Here's how the part is built. I have some questions about the finished solid (model axes, mm). A direction names the side the tool comes from. Give positions to 0.01 mm unless a question says otherwise; leave off trailing zeros. Loops run counter-clockwise (first coordinate to the right, second up) from the corner with the lowest first, then second, coordinate; pieces in that order, holes last.
Q1. For faces 1 (the face through (-0.95, 0.78, -126.09)), 2 (the face through (-0.91, 0.78, -102.55)), which set-ups out of +Z, -Z, +X, -X, +Y, -Y let a thin tool reach every point of the face, with its end or its side?
Q2. If we section it at B-B (x = -76.2): Please give me the cut outline in (y, z), plus the area to 3 significant figures.
Q3. We'd pull the mould along X, two halves only. Please class faces 3 (the face through (-42.125, 0.805, -5.834)), 4 (the face through (-54, 1.588, -63)), 5 (the face through (-87.95, 0.78, -0.91)), 6 (the face through (-37.19, 0.78, -100.65)): +X half, -X half, draft (parallel to the pull), parting line (faces both ways), or undercut.
Q4. If we section it at A-A (z = -63.5): Please give me the cut outline in (x, y).
Q5. I need wall thicknesses on line 1 (Z direction, x = -44.45, y = 0.9); line 2 (X direction, y = 1.2, z = -12.7); line 3 (X direction, y = 1.1, z = -120.65). Which ranges of each line are inside material? Lowest first, please.
Q6. If we section it at C-C (x = -44.45): Please give me the cut outline in (y, z).
Q7. If we section it at D-D (z = -12.7): Please give me the cut outline in (x, y), plus the area to 3 significant figures.
Autodesk Inventor part; units mm, degrees
ref_plane "YZ Plane" through (0, 0, 0) normal (1, 0, 0) x (0, 1, 0)
ref_plane "XZ Plane" through (0, 0, 0) normal (0, 1, 0) x (-1, 0, 0)
ref_plane "XY Plane" through (0, 0, 0) normal (0, 0, 1) x (1, 0, 0)
sketch "Sketch1" plane through (0, 0, 0) normal (0, 1, 0) x (-1, 0, 0)
  line L0 (3.175, 0) -> (85.725, 0)
  line L1 (88.9, -3.175) -> (88.9, -123.825)
  line L2 (85.725, -127) -> (3.175, -127)
  line L3 (0, -123.825) -> (0, -104.775)
  line L4 (3.175, -101.6) -> (34.925, -101.6)
  line L5 (0, -3.175) -> (0, -22.225)
  line L6 (3.175, -25.4) -> (34.925, -25.4)
  line L7 (38.1, -28.575) -> (38.1, -98.425)
  arc A0 (88.9, -3.175) -> (85.725, 0) centre (85.725, -3.175) ccw
  arc A1 (85.725, -127) -> (88.9, -123.825) centre (85.725, -123.825) ccw
  arc A2 (0, -123.825) -> (3.175, -127) centre (3.175, -123.825) ccw
  arc A3 (3.175, -101.6) -> (0, -104.775) centre (3.175, -104.775) ccw
  arc A4 (34.925, -101.6) -> (38.1, -98.425) centre (34.925, -98.425) ccw
  arc A5 (3.175, 0) -> (0, -3.175) centre (3.175, -3.175) ccw
  arc A6 (0, -22.225) -> (3.175, -25.4) centre (3.175, -22.225) ccw
  arc A7 (38.1, -28.575) -> (34.925, -25.4) centre (34.925, -28.575) ccw
  line L8 (0, 0) -> (0, -12.7)
  line L9 (0, 0) -> (0, -12.7)
  line L10 (0, -12.7) -> (12.7, -12.7)
  line L11 (12.7, -12.7) -> (76.2, -12.7)
  line L12 (0, -114.3) -> (12.7, -114.3)
  line L13 (12.7, -114.3) -> (76.2, -114.3)
  line L14 (76.2, -12.7) -> (44.45, -12.7)
  line L15 (44.45, -12.7) -> (44.45, -6.35)
  line L16 (76.2, -114.3) -> (44.45, -114.3)
  line L17 (44.45, -114.3) -> (44.45, -120.65)
  line L18 (44.45, -12.7) -> (44.45, -114.3)
  line L19 (44.45, -63.5) -> (52.1099, -63.5)
  point P0 (88.9, 0)
  point P1 (88.9, -127)
  point P2 (0, -127)
  point P3 (0, -101.6)
  point P4 (38.1, -101.6)
  point P5 (0, -25.4)
  dimension "d0" = 88.9
  dimension "d1" = 127
  dimension "d2" = 25.4
  dimension "d3" = 38.1
  dimension "d4" = 25.4
  dimension "d5" = 3.175
  dimension "d8" = 12.7
  dimension "d10" = 63.5
  dimension "d11" = 31.75
  dimension "d12" = 6.35
extrude "Extrusion1" add sketch "Sketch1" along normal blind 1.5875
hole "Hole1" at (-76.2, 0, -12.7) at (-44.45, 0, -6.35) at (-12.7, 0, -12.7) at (-12.7, 0, -114.3) at (-44.45, 0, -120.65) at (-76.2, 0, -114.3) at (-44.45, 0, -63.5) direction (0, 1, 0) diameter 4.7625 end through all
properties part number "triball holder"
Check sheet entries:
1. face 1: -Z, +X, +Y, -Y
1. face 2: +X, +Y, -Y
2. outline: (0, -127) - (1.59, -127) - (1.59, -116.68) - (0, -116.68) - close; (0, -111.92) - (1.59, -111.92) - (1.59, -15.08) - (0, -15.08) - close; (0, -10.32) - (1.59, -10.32) - (1.59, 0) - (0, 0) - close
2. area: 186 mm2
3. face 3: undercut
3. face 4: draft
3. face 5: -X half
3. face 6: +X half
4. outline: (-88.9, 0) - (-46.83, 0) - (-46.83, 1.59) - (-88.9, 1.59) - close; (-42.07, 0) - (-38.1, 0) - (-38.1, 1.59) - (-42.07, 1.59) - close
5. line 1: z = -127 to -123.03, -118.27 to -65.88, -61.12 to -8.73, -3.97 to 0
5. line 2: x = -88.9 to -78.58, -73.82 to -15.08, -10.32 to 0
5. line 3: x = -88.9 to -46.83, -42.07 to 0
6. outline: (0, -127) - (1.59, -127) - (1.59, -123.03) - (0, -123.03) - close; (0, -118.27) - (1.59, -118.27) - (1.59, -65.88) - (0, -65.88) - close; (0, -61.12) - (1.59, -61.12) - (1.59, -8.73) - (0, -8.73) - close; (0, -3.97) - (1.59, -3.97) - (1.59, 0) - (0, 0) - close
7. outline: (-88.9, 0) - (-78.58, 0) - (-78.58, 1.59) - (-88.9, 1.59) - close; (-73.82, 0) - (-15.08, 0) - (-15.08, 1.59) - (-73.82, 1.59) - close; (-10.32, 0) - (0, 0) - (0, 1.59) - (-10.32, 1.59) - close
7. area: 126 mm2
